```python
from build123d import *
from OCP.BRepFilletAPI import BRepFilletAPI_MakeChamfer
from build123d.topology import SkipClean

# Parameters (mm, degrees)
SKETCH1_R                      = 0.8
BOSS_EXTRUDE1_DEPTH            = 2
FILLET2_R                      = 2.5
SKETCH2_R                      = 3.51040764
BOSS_EXTRUDE2_DEPTH            = 2
BOSS_EXTRUDE3_START            = -2
SKETCH3_R                      = 10.475
BOSS_EXTRUDE3_DEPTH            = 7.6
SKETCH4_R                      = 8.475
CUT_EXTRUDE1_DEPTH             = 2
SKETCH5_R                      = 0.75
BOSS_EXTRUDE4_DEPTH            = 2
CHAMFER1_SIZE2                 = 1.154700538
CHAMFER1_SIZE                  = 2
CIRPATTERN2_COUNT              = 4
CHAMFER1_OF_CIRPATTERN2_SIZE   = 2
CHAMFER1_OF_CIRPATTERN2_SIZE_2 = 1.154700538
SKETCH6_R                      = 0.73
BOSS_EXTRUDE5_DEPTH            = 3.5


with BuildPart() as part:
    # Sketch1 → Boss-Extrude1 (new body)
    with BuildSketch(Plane(origin=(0, 0, 0), x_dir=(0, 1, 0), z_dir=(0, 0, 1))):
        with BuildLine():
            Line((-1.75, 1.75), (-1.75, 6))
            ThreePointArc((-1.75, 6), (0, 7.75), (1.75, 6))
            Line((1.75, 6), (1.75, 1.75))
            Line((1.75, 1.75), (6, 1.75))
            ThreePointArc((6, 1.75), (7.75, 0), (6, -1.75))
            Line((6, -1.75), (1.75, -1.75))
            Line((1.75, -1.75), (1.75, -6))
            ThreePointArc((1.75, -6), (0, -7.75), (-1.75, -6))
            Line((-1.75, -6), (-1.75, -1.75))
            Line((-1.75, -1.75), (-6, -1.75))
            ThreePointArc((-6, -1.75), (-7.75, 0), (-6, 1.75))
            Line((-6, 1.75), (-1.75, 1.75))
        make_face()
        with Locations(Location((0, 6, 0), (0, 0, 270))):
            Circle(SKETCH1_R, mode=Mode.SUBTRACT)
        with Locations(Location((6, 0, 0), (0, 0, 270))):
            Circle(SKETCH1_R, mode=Mode.SUBTRACT)
        with Locations(Location((0, -6, 0), (0, 0, 270))):
            Circle(SKETCH1_R, mode=Mode.SUBTRACT)
        with Locations(Location((-6, 0, 0), (0, 0, 270))):
            Circle(SKETCH1_R, mode=Mode.SUBTRACT)
    extrude(amount=BOSS_EXTRUDE1_DEPTH)

    # Fillet2
    fillet2_edges = [part.edges().sort_by_distance(p)[0] for p in [
        (1.75, 1.75, 1),
        (1.75, -1.75, 1),
        (-1.75, -1.75, 1),
        (-1.75, 1.75, 1),
    ]]
    fillet(fillet2_edges, radius=FILLET2_R)

    # Sketch2 → Boss-Extrude2 (add)
    with BuildSketch(Plane(origin=(0, 0, 0), x_dir=(1, 0, 0), z_dir=(0, 0, -1))):
        with Locations(Location((0, 0, 0), (0, 0, 45))):
            Circle(SKETCH2_R)
    extrude(amount=BOSS_EXTRUDE2_DEPTH)

    # Sketch3 → Boss-Extrude3 (add)
    with BuildSketch(Plane(origin=(0, 0, 0), x_dir=(0, 1, 0), z_dir=(0, 0, 1)).offset(BOSS_EXTRUDE3_START)):
        with Locations(Location((0, 0, 0), (0, 0, 270))):
            Circle(SKETCH3_R)
    extrude(amount=-BOSS_EXTRUDE3_DEPTH)

    # Sketch4 → Cut-Extrude1 (cut)
    with BuildSketch(Plane(origin=(0, 0, -9.6), x_dir=(1, 0, 0), z_dir=(0, 0, -1))):
        with Locations(Location((0, 0, 0), (0, 0, 180))):
            Circle(SKETCH4_R)
    extrude(amount=-CUT_EXTRUDE1_DEPTH, mode=Mode.SUBTRACT)

    # Sketch5 → Boss-Extrude4 (add)
    with BuildSketch(Plane(origin=(0, 0, -9.6), x_dir=(1, 0, 0), z_dir=(0, 0, -1))):
        with BuildLine():
            Line((0, 0), (-4, 0))
            Line((-4, 0), (-2, -10.282296679))
            ThreePointArc((-2, -10.282296679), (-1.004631098, -10.426712874), (0, -10.475))
            Line((0, -10.475), (0, 0))
        make_face()
        with Locations(Location((-1.7, -1.7, 0), (0, 0, 180))):
            Circle(SKETCH5_R, mode=Mode.SUBTRACT)
    boss_extrude4 = extrude(amount=BOSS_EXTRUDE4_DEPTH)

    # Chamfer1
    chamfer1_edges = [part.edges().sort_by_distance(p)[0] for p in [
        (-1.004631098, 10.426712874, -11.6),
    ]]
    chamfer1_side = [part.faces().sort_by_distance(p)[0] for p in [
        (-1.004631098, 10.426712874, -11.576905989),
    ]]
    chamfer(chamfer1_edges, length=CHAMFER1_SIZE - 0.0001, length2=CHAMFER1_SIZE2 - 0.0001, reference=chamfer1_side[0])  # a hair under: the kernel refuses the full size

    # CirPattern2: Boss-Extrude4 ×4 about axis
    with SkipClean():  # the faces are left unmerged after this step: merging them gives an invalid solid
        cirpattern2_axis = Axis((0, 0, 0), (0, 0, 1))
        for i in range(1, CIRPATTERN2_COUNT):
            add(boss_extrude4.rotate(cirpattern2_axis, i * 360 / CIRPATTERN2_COUNT))

    # Chamfer1 of CirPattern2
    chamfer1_of_cirpattern2_edges_1 = [part.edges().sort_by_distance(p)[0] for p in [
        (-10.426712874, -1.004631098, -11.6),
    ]]
    chamfer1_of_cirpattern2_side_1 = [part.faces().sort_by_distance(p)[0] for p in [
        (-10.426712874, -1.004631098, -11.576905989),
    ]]
    chamfer1_of_cirpattern2_edges_2 = [part.edges().sort_by_distance(p)[0] for p in [
        (1.004631098, -10.426712874, -11.6),
    ]]
    chamfer1_of_cirpattern2_side_2 = [part.faces().sort_by_distance(p)[0] for p in [
        (1.004631098, -10.426712874, -11.576905989),
    ]]
    chamfer1_of_cirpattern2_edges_3 = [part.edges().sort_by_distance(p)[0] for p in [
        (10.426712874, 1.004631098, -11.6),
    ]]
    chamfer1_of_cirpattern2_side_3 = [part.faces().sort_by_distance(p)[0] for p in [
        (10.426712874, 1.004631098, -11.576905989),
    ]]
    chamfer1_of_cirpattern2 = BRepFilletAPI_MakeChamfer(part.part.solid().wrapped)
    for e in chamfer1_of_cirpattern2_edges_1:
        chamfer1_of_cirpattern2.Add(CHAMFER1_OF_CIRPATTERN2_SIZE - 0.0001, CHAMFER1_OF_CIRPATTERN2_SIZE_2 - 0.0001, e.wrapped, chamfer1_of_cirpattern2_side_1[0].wrapped)
    for e in chamfer1_of_cirpattern2_edges_2:
        chamfer1_of_cirpattern2.Add(CHAMFER1_OF_CIRPATTERN2_SIZE - 0.0001, CHAMFER1_OF_CIRPATTERN2_SIZE_2 - 0.0001, e.wrapped, chamfer1_of_cirpattern2_side_2[0].wrapped)
    for e in chamfer1_of_cirpattern2_edges_3:
        chamfer1_of_cirpattern2.Add(CHAMFER1_OF_CIRPATTERN2_SIZE - 0.0001, CHAMFER1_OF_CIRPATTERN2_SIZE_2 - 0.0001, e.wrapped, chamfer1_of_cirpattern2_side_3[0].wrapped)
    add(Compound.cast(chamfer1_of_cirpattern2.Shape()), mode=Mode.REPLACE)  # a hair under: the kernel refuses the full size

    # Sketch6 → Boss-Extrude5 (add)
    with BuildSketch(Plane(origin=(0, 0, -11.6), x_dir=(1, 0, 0), z_dir=(0, 0, -1))):
        with Locations(Location((0, 0, 0), (0, 0, 180))):
            Circle(SKETCH6_R)
    extrude(amount=BOSS_EXTRUDE5_DEPTH)


solid = part.part
```
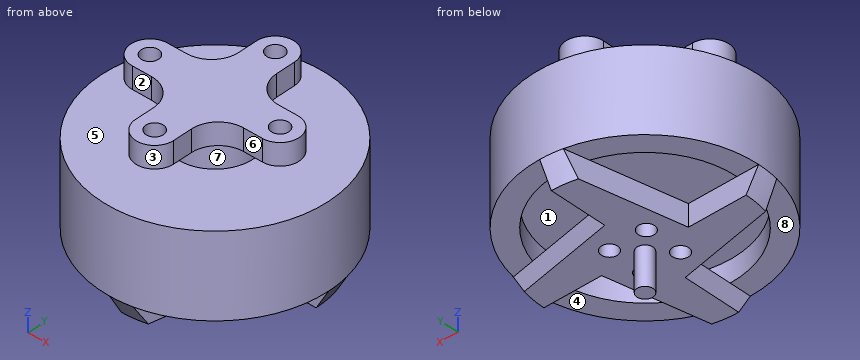
Source: CAD feature listing. Evaluate the final solid. Frame: model axes, mm. Face numbers are marked on the shaded views. A direction names the side the tool comes from. Give positions to 0.01 mm unless a question says otherwise; leave off trailing zeros. Write each loop counter-clockwise with the first axis right and the second up, starting at its lowest first coordinate (ties: lowest second). Pieces come first, ordered by that corner, then holes.
1. First-contact query: pin 1 (6 mm diameter, centred on x = 6.5, z = -3.5, fed in from +Y); pin 2 (4 mm diameter, centred on x = -6, y = -1, fed in from -Z); pin 3 (4 mm diameter, centred on y = 5, z = -3, fed in from +X); pin 4 (8.5 mm diameter, centred on x = -2.5, y = 2.5, fed in from +Z). Flat tips, straight axial feed; report the tip coordinate or a pass-through.
2. Section query A-A (z = 0.5). Return the cut outline in (x, y), then the cut area to 3 significant figures.
3. Access query for the marked faces 1, 2, 3 and 4. Directions: +Z, -Z, +X, -X, +Y, -Y. A direction counts if a zero-diameter tool reaches every point of the face in a straight line with its end or side. Return the directions, or none.
4. Pull-direction query (Z, two-part tool) for the marked faces 5, 6, 7 and 8; classes: +Z half, -Z half, draft (parallel to the pull), parting line (faces both ways), or undercut.
5. Material intervals for line 1 along Y through (x, z) = (0, 0.8); line 2 along Z through (x, y) = (-3.25, -0.25); line 3 along X through (y, z) = (-0.5, 0.5), sorted ascending.
6. Section query C-C (x = -6.5). Return the cut outline in (y, z), then the cut area to 3 significant figures.
7. Section query D-D (z = -9). Return the cut outline in (x, y) (3 decimals), then the cut area to 3 significant figures.
8. Section query B-B (x = -3). Return the cut outline in (y, z).
Output values:
1. pin 1: stops at y = 9.87
1. pin 2: stops at z = -11.6
1. pin 3: stops at x = 10.04
1. pin 4: stops at z = 2
2. outline: (-6, -1.75) - (-4.25, -1.75) arc R2.5 cw to (-1.75, -4.25) - (-1.75, -6) arc R1.75 ccw to (1.75, -6) - (1.75, -4.25) arc R2.5 cw to (4.25, -1.75) - (6, -1.75) arc R1.75 ccw to (6, 1.75) - (4.25, 1.75) arc R2.5 cw to (1.75, 4.25) - (1.75, 6) arc R1.75 ccw to (-1.75, 6) - (-1.75, 4.25) arc R2.5 cw to (-4.25, 1.75) - (-6, 1.75) arc R1.75 ccw to start; hole circle Ø1.6 at (-6, 0); hole circle Ø1.6 at (0, -6); hole circle Ø1.6 at (0, 6); hole circle Ø1.6 at (6, 0)
2. area: 88.3 mm2
3. face 1: none
3. face 2: +Z, -X, -Y
3. face 3: +Z, -Y
3. face 4: -Z, +X, -Y
4. face 5: undercut
4. face 6: draft
4. face 7: undercut
4. face 8: -Z half
5. line 1: y = -7.75 to -6.8, -5.2 to 5.2, 6.8 to 7.75
5. line 2: z = -11.6 to -9.6, -7.6 to 2
5. line 3: x = -7.68 to -6.62, -5.38 to 5.38, 6.62 to 7.68
6. outline: (-8.21, -9.6) - (-5.44, -9.6) - (-5.44, -7.6) - (5.44, -7.6) - (5.44, -9.6) - (8.21, -9.6) - (8.21, -2) - (-8.21, -2) - close; (-2.74, -11.6) - (0, -11.6) - (0, -9.6) - (-2.74, -9.6) - close; (-1.68, 0) - (-0.62, 0) - (-0.62, 2) - (-1.68, 2) - close; (0.62, 0) - (1.68, 0) - (1.68, 2) - (0.62, 2) - close
6. area: 113 mm2
7. outline: circle Ø20.95 at (0, 0); hole circle Ø16.95 at (0, 0)
7. area: 119 mm2
8. outline: (-10.04, -9.6) - (-7.93, -9.6) - (-7.93, -7.6) - (7.93, -7.6) - (7.93, -9.6) - (10.04, -9.6) - (10.04, -2) - (1.82, -2) - (1.82, 0) - (2.08, 0) - (2.08, 2) - (-2.08, 2) - (-2.08, 0) - (-1.82, 0) - (-1.82, -2) - (-10.04, -2) - close; (-3.42, -11.6) - (5.14, -11.6) - (5.14, -9.6) - (-3.42, -9.6) - close
